Check sheet for the modelled part. Datum: model origin and axes. Units: mm. A direction names the side the tool comes from. Round coordinates to 2 decimals unless told otherwise and drop trailing zeros. Loops run counter-clockwise (first coordinate to the right, second up) from the corner with the lowest first, then second, coordinate; pieces in that order, holes last. Notation, with made-up numbers: (36, -19.5) -> (41, -19.5) arc R18 cw to (41, -11.5) -> close; hole circle Ø5 at (80, 47.25). An arc over 180 degrees is marked (long way). One line per question, with ' | ' between items.
```python
from build123d import *

# Parameters (mm, degrees)
F1_DEPTH = 5
F2_R     = 2


with BuildPart() as f1:
    # F0 (on Front) → F1 (new body)
    with BuildSketch(Plane.XZ):
        with BuildLine():
            Line((-8.75, 15.1554445662), (-12.5, 21.6506350946))
            ThreePointArc((-12.5, 21.6506350946), (-21.6506350946, 12.5), (-25, 0))
            Line((-25, 0), (-17.5, 0))
            ThreePointArc((-17.5, 0), (-15.1554445662, 8.75), (-8.75, 15.1554445662))
        make_face()
        with BuildLine():
            Line((-17.5, 0), (-25, 0))
            ThreePointArc((-25, 0), (-21.6506350946, -12.5), (-12.5, -21.6506350946))
            Line((-12.5, -21.6506350946), (-8.75, -15.1554445662))
            ThreePointArc((-8.75, -15.1554445662), (-15.1554445662, -8.75), (-17.5, 0))
        make_face()
        with BuildLine():
            Line((-15, 0), (-17.5, 0))
            ThreePointArc((-17.5, 0), (-15.1554445662, -8.75), (-8.75, -15.1554445662))
            Line((-8.75, -15.1554445662), (-7.5, -12.9903810568))
            ThreePointArc((-7.5, -12.9903810568), (-12.9903810568, -7.5), (-15, 0))
        make_face()
        with BuildLine():
            Line((7.5, 12.9903810568), (8.75, 15.1554445662))
            ThreePointArc((8.75, 15.1554445662), (0, 17.5), (-8.75, 15.1554445662))
            Line((-8.75, 15.1554445662), (-7.5, 12.9903810568))
            ThreePointArc((-7.5, 12.9903810568), (0, 15), (7.5, 12.9903810568))
        make_face()
        with BuildLine():
            Line((8.75, 15.1554445662), (12.5, 21.6506350946))
            ThreePointArc((12.5, 21.6506350946), (0, 25), (-12.5, 21.6506350946))
            Line((-12.5, 21.6506350946), (-8.75, 15.1554445662))
            ThreePointArc((-8.75, 15.1554445662), (0, 17.5), (8.75, 15.1554445662))
        make_face()
        with BuildLine():
            Line((17.5, 0), (25, 0))
            ThreePointArc((25, 0), (21.6506350946, 12.5), (12.5, 21.6506350946))
            Line((12.5, 21.6506350946), (8.75, 15.1554445662))
            ThreePointArc((8.75, 15.1554445662), (15.1554445662, 8.75), (17.5, 0))
        make_face()
        with BuildLine():
            Line((7.5, -12.9903810568), (8.75, -15.1554445662))
            ThreePointArc((8.75, -15.1554445662), (15.1554445662, -8.75), (17.5, 0))
            Line((17.5, 0), (15, 0))
            ThreePointArc((15, 0), (12.9903810568, -7.5), (7.5, -12.9903810568))
        make_face()
        with BuildLine():
            Line((8.75, -15.1554445662), (12.5, -21.6506350946))
            ThreePointArc((12.5, -21.6506350946), (21.6506350946, -12.5), (25, 0))
            Line((25, 0), (17.5, 0))
            ThreePointArc((17.5, 0), (15.1554445662, -8.75), (8.75, -15.1554445662))
        make_face()
    extrude(amount=F1_DEPTH)

    # F2
    f2_edges = [f1.edges().sort_by_distance(p)[0] for p in [
        (7.5, -2.5, 12.990381),
        (-7.5, -2.5, 12.990381),
        (-15, -2.5, 0),
        (-7.5, -2.5, -12.990381),
        (7.5, -2.5, -12.990381),
        (15, -2.5, 0),
        (-12.5, -2.5, -21.650635),
        (12.5, -2.5, -21.650635),
    ]]
    fillet(f2_edges, radius=F2_R)


solid = f1.part
```
(1) Sectioned sample at C-C, the plane z = 5. Record the cut outline in (x, y).
Answer:
outline: (-24.49, -5) -> (-16.77, -5) -> (-16.77, 0) -> (-24.49, 0) -> close; (16.77, -5) -> (24.49, -5) -> (24.49, 0) -> (16.77, 0) -> close
(2) Scan lines: probe 1 along Z at (x, y) = (11.5, -3); probe 2 along X at (y, z) = (-1.4, -7); probe 3 along X at (y, z) = (-3.5, 9.5). Record each from-to range of solid material in increasing order.
Answer:
probe 1: z = -19.92 to -9.63, 13.19 to 22.2 | probe 2: x = -24 to -13.27, 13.27 to 24 | probe 3: x = -23.12 to -14.7, 14.7 to 23.12
(3) Go/stop test with flat-tipped pins: pin 1 (2 mm diameter, centred on x = 11.5, y = -3, fed in from +Z); pin 2 (0.5 mm diameter, centred on x = -17, y = -1.5, fed in from +Z); pin 3 (1.5 mm diameter, centred on y = -3, z = -2.5, fed in from +X). Record where each tip stops, or that it passes through.
Answer:
pin 1: stops at z = 22.69 | pin 2: stops at z = 18.56 | pin 3: stops at x = 24.94
(4) Sectioned sample at D-D, the plane x = -20. Record the cut outline in (y, z), and give its area (3 significant figures).
Answer:
outline: (-5, -15) -> (0, -15) -> (0, 15) -> (-5, 15) -> close | area: 150 mm2
(5) Sectioned sample at A-A, the plane z = -6. Record the cut outline in (x, y).
Answer:
outline: (-24.27, -5) -> (-13.75, -5) -> (-13.75, 0) -> (-24.27, 0) -> close; (13.75, -5) -> (24.27, -5) -> (24.27, 0) -> (13.75, 0) -> close
(6) Set-up check for faces 5 (the face through (0, -5, 18)), 6 (the face through (-15.538, -2.535, -0.518)): record each of +Z, -Z, +X, -X, +Y, -Y from which the full face is reachable in a straight line by a thin tool's end or side.
Answer:
face 5: +Z, -Z, +X, -X, -Y | face 6: +Y, -Y
(7) Sectioned sample at B-B, the plane y = -3.4. Record the cut outline in (x, z), and give its area (3 significant figures).
Answer:
outline: (-17.5, 0) arc R17.5 cw to (-8.75, 15.16) -> (-8.44, 14.62) arc R2 ccw to (-5.92, 13.78) arc R15 cw to (5.92, 13.78) arc R2 ccw to (8.44, 14.62) -> (8.75, 15.16) arc R17.5 cw to (17.5, 0) -> (16.88, 0) arc R2 ccw to (14.9, -1.76) arc R15 cw to (8.98, -12.02) arc R2 ccw to (8.44, -14.62) -> (11.46, -19.84) arc R2 ccw to (14.34, -20.48) arc R25 ccw (long way) to (-14.34, -20.48) arc R2 ccw to (-11.46, -19.84) -> (-8.44, -14.62) arc R2 ccw to (-8.98, -12.02) arc R15 cw to (-14.9, -1.76) arc R2 ccw to (-16.88, 0) -> close | area: 956 mm2
(8) Mould release check, pull along Z, two halves, no side actions. Record for faces 1 (the face through (15.09, -2.46, 8.86)), 2 (the face through (12.73, -2.54, -20.79)), 3 (the face through (-8.21, -2.54, -13.24)), 4 (the face through (0, 0, 18)): +Z half, -Z half, draft (parallel to the pull), parting line (faces both ways), or undercut.
Answer:
face 1: undercut | face 2: -Z half | face 3: undercut | face 4: draft
